The listing builds one solid part. Answer for the finished solid, in the listing's coordinates (mm). A direction names the side the tool comes from. Give positions to 0.01 mm unless a question says otherwise; leave off trailing zeros. Loops run counter-clockwise (first coordinate to the right, second up) from the corner with the lowest first, then second, coordinate; pieces in that order, holes last. Notation, with made-up numbers: M 76.25,60 L 126.25,60 A24 ccw 126.25,84 Z; hole C -17,-16.5 d2. An arc over 180 degrees is marked long. Return JSON: item names as keys, results as strings.
from build123d import *

# Parameters (mm, degrees)
F0_R     = 2.45
F0_R_2   = 1.45
F1_DEPTH = 2.5
F2_DEPTH = 2
F3_DEPTH = 3.5


# Not quite as in the source:
# - a feature names something its author has since deleted; it is built from what else it names


with BuildPart() as f1:
    # F0 (on Top) → F1 (new body)
    with BuildSketch(Plane.XY):
        Circle(F0_R)
        Circle(F0_R_2, mode=Mode.SUBTRACT)
    extrude(amount=F1_DEPTH)

    # F2 (add): a face of the model
    f2_faces = [f1.faces().sort_by_distance(p)[0] for p in [
        (-2.3807035354, 0, 2.5),
    ]]
    extrude(f2_faces, amount=F2_DEPTH)

    # F0 (on Top) → F3 (join)
    with BuildSketch(Plane.XY):
        Polygon((3.25, -1.8763883749), (3.25, 1.8763883749), (0, 3.7527767497), (-3.25, 1.8763883749), (-3.25, -1.8763883749), (0, -3.7527767497), align=None)
        Circle(F0_R, mode=Mode.SUBTRACT)
    extrude(amount=F3_DEPTH)


solid = f1.part
(1) A tool of negligible diameter and unlimited length cuts with its end or side. For faces 1 (the flat face through (1.6, -2.83, 1.73)), 2 (the flat face through (0, 3, 3.5)), from which of +Z, -Z, +X, -X, +Y, -Y can it reach the whole face along a straight path? Write none if from no direction.
Values follow:
{"face 1": "+Z, -Z, +X, -Y", "face 2": "+Z"}
(2) Determine the mould class of faces 3 (the cylindrical face through (-1.45, 0.06, 2.22)), 4 (the flat face through (3.25, 0, 2)), 5 (the flat face through (-1.6, 2.83, 1.73)) for opening direction X: released by +X, released by -X, zero draft, split by the parting line, or undercut.
Values follow:
{"face 3": "undercut", "face 4": "released by +X", "face 5": "released by -X"}
(3) The part is cut by section C-C (x = -0.5). Determine the outline of the cut face in (y, z), and give its area (3 significant figures).
Values follow:
{"outline": "M -3.46,0 L -1.36,0 L -1.36,4.5 L -2.4,4.5 L -2.4,3.5 L -3.46,3.5 Z; M 1.36,0 L 3.46,0 L 3.46,3.5 L 2.4,3.5 L 2.4,4.5 L 1.36,4.5 Z", "area": "16.8 mm²"}
(4) The part is cut by section B-B (z = 2.4). Determine the outline of the cut face in (x, y), and give its area (3 significant figures).
Values follow:
{"outline": "M -3.25,-1.88 L 0,-3.75 L 3.25,-1.88 L 3.25,1.88 L 0,3.75 L -3.25,1.88 Z; hole C 0,0 d2.9", "area": "30.0 mm²"}
(5) The part is cut by section D-D (y = 1.75). Determine the outline of the cut face in (x, z), and give its area (3 significant figures).
Values follow:
{"outline": "M -3.25,0 L 3.25,0 L 3.25,3.5 L 1.71,3.5 L 1.71,4.5 L -1.71,4.5 L -1.71,3.5 L -3.25,3.5 Z", "area": "26.2 mm²"}
(6) The part is cut by section A-A (y = 0). Determine the outline of the cut face in (x, z).
Values follow:
{"outline": "M -3.25,0 L -1.45,0 L -1.45,4.5 L -2.45,4.5 L -2.45,3.5 L -3.25,3.5 Z; M 1.45,0 L 3.25,0 L 3.25,3.5 L 2.45,3.5 L 2.45,4.5 L 1.45,4.5 Z"}
(7) Straight lines are drawn through the part: line 1 along Z through (x, y) = (0.75, 2.75); line 2 along Y through (x, z) = (-0.25, 0.75); line 3 along X through (y, z) = (-0.25, 1.3). For each, find the intervals that lie inside material, in ascending order.
Values follow:
{"line 1": "0 to 3.5", "line 2": "-3.61 to -1.43, 1.43 to 3.61", "line 3": "-3.25 to -1.43, 1.43 to 3.25"}
(8) Given pin 1 (3.5 mm diameter, centred on x = 0, y = 0, fed in from -Z), flat-ended and moving along its own axis, determine where the tip first touches the part or whether it passes through.
Values follow:
{"pin 1": "z = 0"}
